```python
from build123d import *

# Parameters (mm, degrees)
SKETCH1_W           = 62.992
SKETCH1_H           = 24.13
BOSS_EXTRUDE1_DEPTH = 8.89
SHELL1_T            = 2.032
SKETCH2_W           = 6.35
SKETCH2_H           = 5.842
CUT_EXTRUDE1_DEPTH  = 8.89
SKETCH3_W           = 6.35
SKETCH3_H           = 8.382
CUT_EXTRUDE2_DEPTH  = 8.89
FILLET1_R           = 2.54
SKETCH4_W           = 90.17
SKETCH4_H           = 31.75
SKETCH4_R           = 1.5
BOSS_EXTRUDE2_DEPTH = 2.032
SKETCH5_W           = 62.992
SKETCH5_H           = 24.13
CUT_EXTRUDE3_DEPTH  = 10.922
FILLET2_R           = 1.27
SKETCH6_W           = 50.8
SKETCH6_H           = 16.51
CUT_EXTRUDE4_DEPTH  = 10.922
FILLET3_R           = 1.27
SKETCH8_W           = 3.302
SKETCH8_H           = 6.35
CUT_EXTRUDE5_DEPTH  = 10.922


with BuildPart() as part:
    # Sketch1 → Boss-Extrude1 (new body)
    with BuildSketch(Plane(origin=(0, 0, 0), x_dir=(1, 0, 0), z_dir=(0, 1, 0))):
        Rectangle(SKETCH1_W, SKETCH1_H)
    extrude(amount=BOSS_EXTRUDE1_DEPTH)

    # Shell1
    shell1_openings = [part.faces().sort_by_distance(p)[0] for p in [
        (0, 0, 0),
    ]]
    offset(amount=SHELL1_T, openings=shell1_openings, kind=Kind.INTERSECTION)

    # Sketch2 → Cut-Extrude1 (cut)
    with BuildSketch(Plane.ZY.offset(33.528)):
        with Locations((0, 2.921)):
            Rectangle(SKETCH2_W, SKETCH2_H)
    extrude(amount=-CUT_EXTRUDE1_DEPTH, mode=Mode.SUBTRACT)

    # Sketch3 → Cut-Extrude2 (cut)
    with BuildSketch(Plane(origin=(33.528, 0, 0), x_dir=(0, 0, -1), z_dir=(1, 0, 0))):
        with Locations((0, 4.191)):
            Rectangle(SKETCH3_W, SKETCH3_H)
    extrude(amount=-CUT_EXTRUDE2_DEPTH, mode=Mode.SUBTRACT)

    # Fillet1
    fillet1_edges = [part.edges().sort_by_distance(p)[0] for p in [
        (-32.512, 5.842, 3.175),
        (-32.512, 5.842, -3.175),
        (32.512, 8.382, -3.175),
        (32.512, 8.382, 3.175),
    ]]
    fillet(fillet1_edges, radius=FILLET1_R)

    # Sketch4 → Boss-Extrude2 (add)
    with BuildSketch(Plane.XZ):
        Rectangle(SKETCH4_W, SKETCH4_H)
        with Locations(Location((-39.878, 7.62, 0), (0, 0, 270))):
            Circle(SKETCH4_R, mode=Mode.SUBTRACT)
        with Locations(Location((-39.878, -7.62, 0), (0, 0, 90))):
            Circle(SKETCH4_R, mode=Mode.SUBTRACT)
        with Locations(Location((39.878, -7.62, 0), (0, 0, 270))):
            Circle(SKETCH4_R, mode=Mode.SUBTRACT)
        with Locations(Location((39.878, 7.62, 0), (0, 0, 90))):
            Circle(SKETCH4_R, mode=Mode.SUBTRACT)
    extrude(amount=BOSS_EXTRUDE2_DEPTH)

    # Sketch5 → Cut-Extrude3 (cut)
    with BuildSketch(Plane.XZ.offset(2.032)):
        Rectangle(SKETCH5_W, SKETCH5_H)
    extrude(amount=-CUT_EXTRUDE3_DEPTH, mode=Mode.SUBTRACT)

    # Fillet2
    fillet2_edges = [part.edges().sort_by_distance(p)[0] for p in [
        (45.085, -1.016, -15.875),
        (45.085, -1.016, 15.875),
        (-45.085, -1.016, 15.875),
        (-45.085, -1.016, -15.875),
        (-33.528, 10.922, 0),
        (0, 10.922, 14.097),
        (33.528, 10.922, 0),
        (33.528, 5.461, 14.097),
        (-33.528, 5.461, 14.097),
        (-33.528, 5.461, -14.097),
        (33.528, 5.461, -14.097),
        (0, 10.922, -14.097),
    ]]
    fillet(fillet2_edges, radius=FILLET2_R)
    fillet2_2_edges = [part.edges().sort_by_distance(p)[0] for p in [
        (-33.528, 0, 8.001),
        (0, 0, 14.097),
        (33.528, 0, -8.001),
        (-33.528, 0, -8.001),
        (0, 0, -14.097),
        (33.528, 0, 8.001),
        (33.156025612, 0, 13.725025612),
        (-33.156025612, 0, -13.725025612),
        (33.156025612, 0, -13.725025612),
        (-33.156025612, 0, 13.725025612),
    ]]
    fillet(fillet2_2_edges, radius=FILLET2_R)

    # Sketch6 → Cut-Extrude4 (cut)
    with BuildSketch(Plane(origin=(0, 10.922, 0), x_dir=(1, 0, 0), z_dir=(0, 1, 0))):
        Rectangle(SKETCH6_W, SKETCH6_H)
    extrude(amount=-CUT_EXTRUDE4_DEPTH, mode=Mode.SUBTRACT)

    # Fillet3
    fillet3_edges = [part.edges().sort_by_distance(p)[0] for p in [
        (25.4, 9.906, -8.255),
        (25.4, 9.906, 8.255),
        (-25.4, 9.906, 8.255),
        (-25.4, 9.906, -8.255),
        (25.4, 10.922, 0),
        (0, 10.922, -8.255),
        (-25.4, 10.922, 0),
        (0, 10.922, 8.255),
    ]]
    fillet(fillet3_edges, radius=FILLET3_R)

    # Sketch8 → Cut-Extrude5 (cut)
    with BuildSketch(Plane(origin=(0, 0, 0), x_dir=(1, 0, 0), z_dir=(0, 1, 0))):
        with Locations((-33.147, 0)):
            Rectangle(SKETCH8_W, SKETCH8_H)
        with Locations((33.147, 0)):
            Rectangle(SKETCH8_W, SKETCH8_H)
    extrude(amount=-CUT_EXTRUDE5_DEPTH, mode=Mode.SUBTRACT)


solid = part.part
```
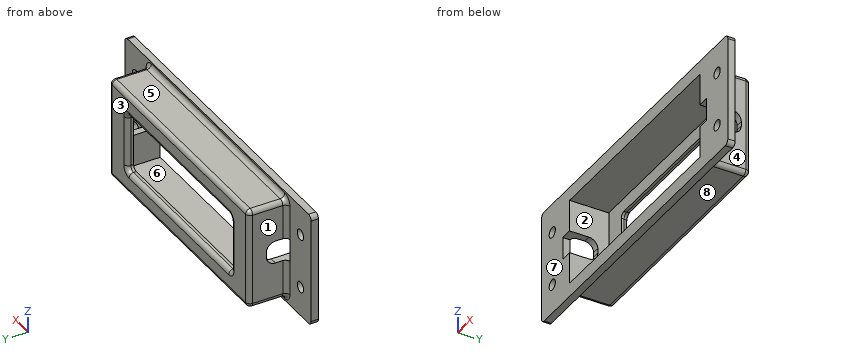
Can you work these out from the model? Positions are in its coordinate system, mm. Face numbers are marked on the shaded views. A direction names the side the tool comes from. Give positions to 0.01 mm unless a question says otherwise; leave off trailing zeros. Order: outer loops, then holes, each group sorted by start corner. A loop starts at its lowest first (then second) coordinate and runs counter-clockwise, first axis right, second up. Notation, with made-up numbers: M -17,78 L 3,78 A11 ccw 3,89 Z; hole C -25.75,13.5 d9. An arc over 180 degrees is marked long. One line per item, written item: value.
1) I want a section at B-B, the plane y = 2.5. List the corners of the cut face in (x, z) for me (3 decimals), plus the area to 3 significant figures.
Answer sheet:
outline: M -33.528,-12.827 A1.27 ccw -32.258,-14.097 L 32.258,-14.097 A1.27 ccw 33.528,-12.827 L 33.528,-3.175 L 31.496,-3.175 L 31.496,-12.065 L -31.496,-12.065 L -31.496,-3.175 L -33.528,-3.175 Z; M -33.528,3.175 L -31.496,3.175 L -31.496,12.065 L 31.496,12.065 L 31.496,3.175 L 33.528,3.175 L 33.528,12.827 A1.27 ccw 32.258,14.097 L -32.258,14.097 A1.27 ccw -33.528,12.827 Z
area: 343 mm^2
2) For P1, Ø1.7, axis at x = -34, y = 2, coming from the +Z side; P2, Ø5, axis at y = 3.5, z = 0.5, coming from the -X side; P3, Ø1, axis at x = 33.5, y = 3.5, coming from the +Z side; P4, Ø10, axis at x = 26, z = 2, coming from the +Y side, each with a flat end and sliding along its axis, tell me the tip position at first contact or that it passes through.
Answer sheet:
P1: stops at z = 13.73
P2: stops at x = -33.53
P3: stops at z = 13.86
P4: stops at y = 10.92
3) On a 3-axis mill with a long thin cutter (end or side, diameter ignored), from which of +Z, -Z, +X, -X, +Y, -Y can I reach the whole of each face in a straight line? I mean the marked faces 1, 2, 3 and 4. Say none if no direction works.
Answer sheet:
face 1: +Z, -Z, -X, +Y
face 2: -Y
face 3: +Z, -Z, +X, -X, +Y
face 4: +Z, -Z, +X, +Y
4) Please list where these lines run through material, in increasing order: line 1 along X through (y, z) = (-1.4, 7.62) (3 decimals); line 2 along X through (y, z) = (4.5, -11.5); line 3 along Z through (x, y) = (-26, 4.75) (3 decimals).
Answer sheet:
line 1: x = -45.085 to -41.378, -38.378 to -31.496, 31.496 to 38.378, 41.378 to 45.085
line 2: x = -33.53 to -31.5, 31.5 to 33.53
line 3: z = -14.097 to -12.065, 12.065 to 14.097
5) We'd pull the mould along Z, two halves only. Please class the marked faces 5, 6, 7 and 8: released by +Z, released by -Z, zero draft, split by the parting line, or undercut.
Answer sheet:
face 5: released by +Z
face 6: undercut
face 7: zero draft
face 8: released by -Z
6) I want a section at A-A, the plane x = 17. List the corners of the cut face in (y, z) for me (3 decimals).
Answer sheet:
outline: M -2.032,-15.875 L 0,-15.875 L 0,-15.367 A1.27 cw 1.27,-14.097 L 9.652,-14.097 A1.27 ccw 10.922,-12.827 L 10.922,-9.525 A1.27 ccw 9.652,-8.255 L 8.89,-8.255 L 8.89,-12.065 L -2.032,-12.065 Z; M -2.032,12.065 L 8.89,12.065 L 8.89,8.255 L 9.652,8.255 A1.27 ccw 10.922,9.525 L 10.922,12.827 A1.27 ccw 9.652,14.097 L 1.27,14.097 A1.27 cw 0,15.367 L 0,15.875 L -2.032,15.875 Z
7) I want a section at C-C, the plane z = 4. List the corners of the cut face in (x, y) for me (3 decimals).
Answer sheet:
outline: M -45.085,-2.032 L -31.496,-2.032 L -31.496,8.89 L -25.4,8.89 L -25.4,9.652 A1.27 ccw -26.67,10.922 L -32.258,10.922 A1.27 ccw -33.528,9.652 L -33.528,1.27 A1.27 cw -34.798,0 L -45.085,0 Z; M 25.4,8.89 L 31.496,8.89 L 31.496,-2.032 L 45.085,-2.032 L 45.085,0 L 34.798,0 A1.27 cw 33.528,1.27 L 33.528,9.652 A1.27 ccw 32.258,10.922 L 26.67,10.922 A1.27 ccw 25.4,9.652 Z
8) I want a section at D-D, the plane z = -11. List the corners of the cut face in (x, y) for me (3 decimals).
Answer sheet:
outline: M -45.085,-2.032 L -31.496,-2.032 L -31.496,8.89 L 31.496,8.89 L 31.496,-2.032 L 45.085,-2.032 L 45.085,0 L 34.798,0 A1.27 cw 33.528,1.27 L 33.528,9.652 A1.27 ccw 32.258,10.922 L -32.258,10.922 A1.27 ccw -33.528,9.652 L -33.528,1.27 A1.27 cw -34.798,0 L -45.085,0 Z
